Can you work these out from the model? Positions are in its coordinate system, mm. A direction names the side the tool comes from. Give positions to 0.01 mm unless a question says otherwise; leave off trailing zeros. Loops run counter-clockwise (first coordinate to the right, second up) from the corner with the lowest first, then second, coordinate; pieces in that order, holes last. Notation, with made-up numbers: (61.25, 38.5) -> (92.25, 38.5) arc R16 ccw to (92.25, 42.5) -> close; hole circle Ø2 at (61.25, 60.25). An arc over 180 degrees is marked (long way). One line per question, with ' | ' between items.
Solid Edge part; units mm, degrees
sketch "Sketch1" plane through (0, 0, 0) normal (0, -1, 0) x (1, 0, 0)
  line L0 (8.6, 31.5) -> (8.6, 7.5)
  line L1 (8.6, 7.5) -> (4, 7.5)
  line L2 (4, 7.5) -> (4, 31.5)
  line L3 (4, 31.5) -> (0, 31.5)
  line L4 (0, 31.5) -> (0, 0)
  line L5 (0, 0) -> (12.6, 0)
  line L6 (12.6, 0) -> (12.6, 31.5)
  line L7 (12.6, 31.5) -> (8.6, 31.5)
extrude "Protrusion1" add sketch "Sketch1" along normal blind 10
sketch "Sketch2" plane through (12.6, -5, 7.5) normal (1, 0, 0) x (0, 1, 0)
  circle A0 centre (0, 20) radius 1.9
extrude "Cutout1" cut sketch "Sketch2" against normal through all
sketch "Sketch3" plane through (6.3, -5, 0) normal (0, 0, -1) x (1, 0, 0)
  line L0 (-6.3, -5) -> (-11.8616, -2.2393)
  line L1 (-6.3, 5) -> (-11.8616, 2.2393)
  line L2 (-6.3, 5) -> (6.3, 5)
  line L3 (6.3, 5) -> (11.8616, 2.2393)
  line L4 (6.3, -5) -> (11.8616, -2.2393)
  line L5 (-6.3, -5) -> (6.3, -5)
  arc A0 (-11.8616, -2.2393) -> (-11.8616, 2.2393) centre (-10.75, 0) cw
  arc A1 (11.8616, 2.2393) -> (11.8616, -2.2393) centre (10.75, 0) cw
  circle A2 centre (-10.75, 0) radius 0.875
  circle A3 centre (10.75, 0) radius 0.875
extrude "ExtrudedProtrusion_4" add sketch "Sketch3" along normal blind 2.5
sketch "Sketch4" plane through (6.3, -10, 8) normal (0, -1, 0) x (0, 0, -1)
  circle A0 centre (4.25, 0) radius 1.6
extrude "ExtrudedCutout_2" cut sketch "Sketch4" against normal blind 5
Q1. On a 3-axis mill with a long thin cutter (end or side, diameter ignored), from which of +Z, -Z, +X, -X, +Y, -Y can I reach the whole of each face in a straight line? I mean faces 1 (the face through (15, -5, 0)), 2 (the face through (3.6, 0, 14.7)), 3 (the face through (8.6, -5, 20)), 4 (the face through (0, -5, 16)). Say none if no direction works.
Entries:
face 1: +Z, +X, +Y, -Y | face 2: +Z, -Z, +X, -X, +Y | face 3: +Z, +Y, -Y | face 4: +Z, -X, +Y, -Y
Q2. If we section it at A-A (z = 27.5): Write out the boundary of the cut face in (x, y), plus the area to 3 significant figures.
Entries:
outline: (0, -10) -> (4, -10) -> (4, -6.9) -> (0, -6.9) -> close; (0, -3.1) -> (4, -3.1) -> (4, 0) -> (0, 0) -> close; (8.6, -10) -> (12.6, -10) -> (12.6, -6.9) -> (8.6, -6.9) -> close; (8.6, -3.1) -> (12.6, -3.1) -> (12.6, 0) -> (8.6, 0) -> close | area: 49.6 mm²
Q3. If we section it at C-C (x = 10): Write out the boundary of the cut face in (y, z).
Entries:
outline: (-10, -2.5) -> (0, -2.5) -> (0, 31.5) -> (-10, 31.5) -> close; hole circle Ø3.8 at (-5, 27.5)
Q4. If we mould it in two halves opening along Z, with no side actions, what happens to faces 5 (the face through (2.028, -5.247, 29.384)), 6 (the face through (-6.95, -4.96, -1.23)), 7 (the face through (6, -5, -2.5)), 8 (the face through (4.74, -7.54, 4.1))? For each: pulls with the +Z half, pulls with the -Z half, needs draft (parallel to the pull), parting line crosses it, or undercut.
Entries:
face 5: undercut | face 6: needs draft | face 7: pulls with the -Z half | face 8: undercut
Q5. For pin 1 Ø3 at (x, y) = (14.5, -6) entering from +Z; pin 2 Ø3 at (y, z) = (-4.5, 17.5) entering from +X; pin 3 Ø1.4 at (x, y) = (7, -6) entering from +Z; pin 4 Ø4 at (x, z) = (6.3, 3.75) entering from +Y, each with a flat end and sliding along its axis, tell me the tip position at first contact or that it passes through.
Entries:
pin 1: z = 0 | pin 2: x = 12.6 | pin 3: z = 7.5 | pin 4: y = 0
Q6. If we section it at D-D (z = 16): Write out the boundary of the cut face in (x, y).
Entries:
outline: (0, -10) -> (4, -10) -> (4, 0) -> (0, 0) -> close; (8.6, -10) -> (12.6, -10) -> (12.6, 0) -> (8.6, 0) -> close
Q7. If we section it at B-B (y = -4.5): Write out the boundary of the cut face in (x, z).
Entries:
outline: (-6.9, -2.5) -> (-5.17, -2.5) -> (-5.17, 0) -> (-6.9, 0) -> close; (-3.73, -2.5) -> (16.33, -2.5) -> (16.33, 0) -> (12.6, 0) -> (12.6, 25.67) -> (8.6, 25.67) -> (8.6, 7.5) -> (4, 7.5) -> (4, 25.67) -> (0, 25.67) -> (0, 0) -> (-3.73, 0) -> close; (0, 29.33) -> (4, 29.33) -> (4, 31.5) -> (0, 31.5) -> close; (8.6, 29.33) -> (12.6, 29.33) -> (12.6, 31.5) -> (8.6, 31.5) -> close; (17.77, -2.5) -> (19.5, -2.5) -> (19.5, 0) -> (17.77, 0) -> close
Q8. If I drill on probe 1 along X at (y, z) = (-3, 26); probe 2 along Z at (x, y) = (1, -5); probe 3 along X at (y, z) = (-5, -0.5) (3 decimals), over which ranges is the centre line in solid material (lowest first)? Write a range as from..to.
Entries:
probe 1: 0..4, 8.6..12.6 | probe 2: -2.5..25.6, 29.4..31.5 | probe 3: -6.95..-5.325, -3.575..16.175, 17.925..19.55
